Here's the drawing with two shaded views (mm, measured from the low corner). I have some questions. A direction names the side the tool comes from. Give positions to 0.01 mm unless a question says otherwise; leave off trailing zeros. Loops run counter-clockwise (first coordinate to the right, second up) from the corner with the lowest first, then second, coordinate; pieces in that order, holes last. Notation, with made-up numbers: M -33.5,38.25 L -19.5,38.25 A33 cw -19.5,66.25 Z; hole C 40.5,71.5 d6. An arc over 180 degrees is marked long. Write item = value, one per line. Start each with the question number.
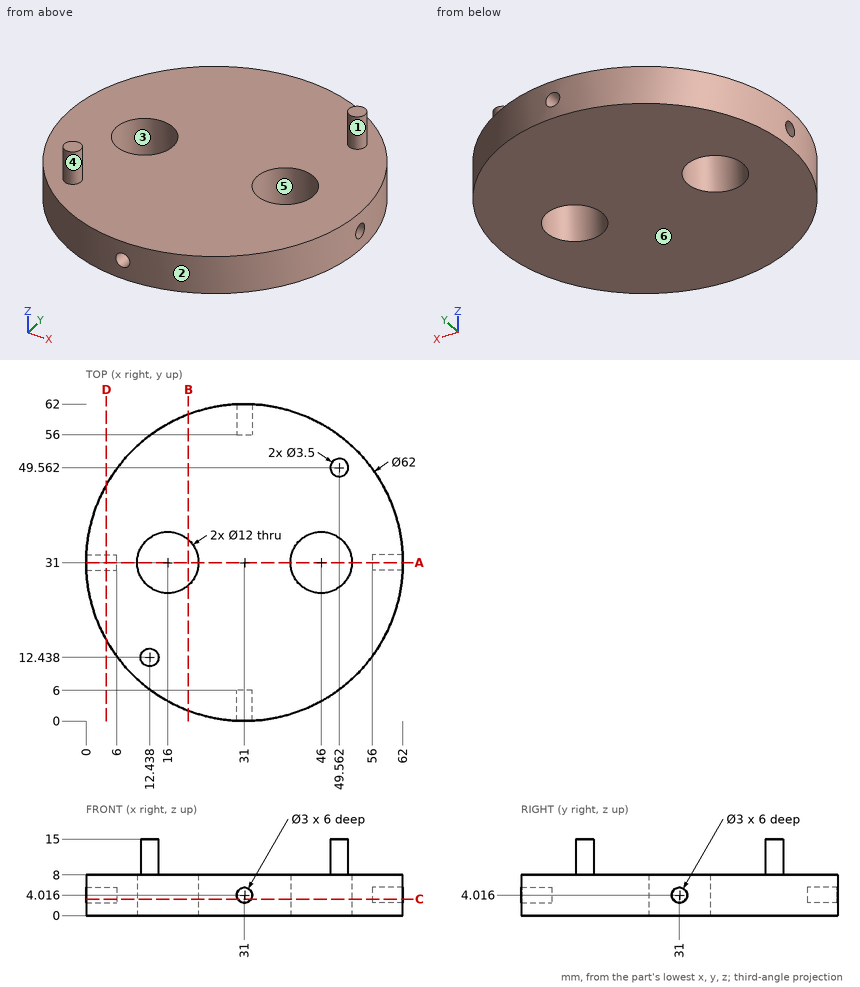
Q1. We'd pull the mould along X, two halves only. Please class the marked faces 3, 4, 5 and 6: pulls with the +X half, pulls with the -X half, needs draft (parallel to the pull), parting line crosses it, or undercut.
Q2. If we section it at C-C, the plane z = 3.25: List the corners of the cut face in (x, y) for me.
Q3. If we section it at B-B, the plane x = 20: List the corners of the cut face in (y, z) for me, then the cut area to 3 significant figures.
Q4. Will these pins go through, and if not, where does the flat tip stop? pin 1 (6 mm diameter, centred on y = 15.5, z = 2.5, fed in from +X); pin 2 (1.8 mm diameter, centred on x = 31, z = 4.02, fed in from -Y); pin 3 (6 mm diameter, centred on x = 35.5, z = 7, fed in from +Y).
Q5. If we section it at D-D, the plane x = 4: List the corners of the cut face in (y, z) for me.
Q6. If I drill on line 1 along X through (y, z) = (31, 2.75); line 2 along Z through (x, y) = (25.5, 27); line 3 along Y through (x, z) = (51, 7.25) (1 decimal), over which ranges is the centre line in solid material (lowest first)?
Q7. On a 3-axis mill with a long thin cutter (end or side, diameter ignored), from which of +Z, -Z, +X, -X, +Y, -Y can I reach the whole of each face in a straight line? I mean the marked faces 1 and 2. Say none if no direction works.
Q8. If we section it at A-A, the plane y = 31: List the corners of the cut face in (x, z) for me, then the cut area to 3 significant figures.
Resolved:
q1.face_3 = undercut
q1.face_4 = parting line crosses it
q1.face_5 = undercut
q1.face_6 = needs draft
q2.outline = M 0.03,29.71 A31 ccw 29.71,0.03 L 29.71,6 L 32.29,6 L 32.29,0.03 A31 ccw 61.97,29.71 L 56,29.71 L 56,32.29 L 61.97,32.29 A31 ccw 32.29,61.97 L 32.29,56 L 29.71,56 L 29.71,61.97 A31 ccw 0.03,32.29 L 6,32.29 L 6,29.71 Z; hole C 16,31 d12; hole C 46,31 d12
q3.outline = M 2.02,0 L 26.53,0 L 26.53,8 L 2.02,8 Z; M 35.47,0 L 59.98,0 L 59.98,8 L 35.47,8 Z
q3.area = 392 mm²
q4.pin_1 = 59.37
q4.pin_2 = 6
q4.pin_3 = 61.96
q5.outline = M 15.77,0 L 46.23,0 L 46.23,8 L 15.77,8 Z; hole C 31,4.02 d3
q6.line_1 = 6 to 10, 22 to 40, 52 to 56
q6.line_2 = 0 to 8
q6.line_3 = 7.3 to 27.7, 34.3 to 54.7
q7.face_1 = +Z
q7.face_2 = +Z, -Z
q8.outline = M 0,0 L 10,0 L 10,8 L 0,8 L 0,5.52 L 6,5.52 L 6,2.52 L 0,2.52 Z; M 22,0 L 40,0 L 40,8 L 22,8 Z; M 52,0 L 62,0 L 62,2.52 L 56,2.52 L 56,5.52 L 62,5.52 L 62,8 L 52,8 Z
q8.area = 268 mm²
